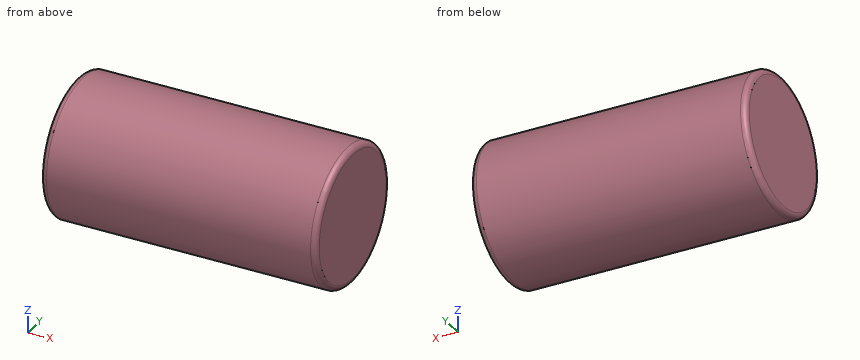
```python
from build123d import *

# Parameters (mm, degrees)
F0_R          = 76.09774
F1_DEPTH      = 152.4
F1_DEPTH_BACK = 152.4
F2_R          = 6.35
F3_R          = 6.35


with BuildPart() as f1:
    # F0 (on Right) → F1 (new body, two sides)
    with BuildSketch(Plane.YZ) as f1_sk:
        Circle(F0_R)
    extrude(amount=F1_DEPTH)
    extrude(f1_sk.sketch, amount=-F1_DEPTH_BACK)

    # F2
    f2_edges = [f1.edges().sort_by_distance(p)[0] for p in [
        (152.4, -76.09774, 0),
    ]]
    fillet(f2_edges, radius=F2_R)

    # F3
    f3_edges = [f1.edges().sort_by_distance(p)[0] for p in [
        (-152.4, -76.09774, 0),
    ]]
    fillet(f3_edges, radius=F3_R)


solid = f1.part
```
Can you work these out from the model? Positions are in its coordinate system, mm. Round coordinates to 2 decimals unless told otherwise and drop trailing zeros. Loops run counter-clockwise (first coordinate to the right, second up) from the corner with the lowest first, then second, coordinate; pieces in that order, holes last. Notation, with made-up numbers: M 73.25,53 L 101.25,53 A8 cw 101.25,63 Z; hole C 87.5,65.25 d8. An arc over 180 degrees is marked long. Answer as a JSON object with one key per item and string values. Group by question number.
Q1. Please list where these lines run through material, in increasing order: L1, parallel to Y at x = 84, z = -2; L2, parallel to Z at x = 37, y = 51.
Q2. Imagine slicing it at A-A, the plane x = -111.5. Please give me the cut outline in (y, z), then the cut area to 3 significant figures.
Q3. Will these pins go through, and if not, where does the flat tip stop? pin 1 (3 mm diameter, centred on x = 26.5, z = 39, fed in from -Y); pin 2 (1 mm diameter, centred on x = 118, z = -42.5, fed in from -Y); pin 3 (4 mm diameter, centred on x = 18.5, z = -37.5, fed in from -Y).
Findings:
{
 "1": {"L1": "y = -76.07 to 76.07", "L2": "z = -56.48 to 56.48"},
 "2": {"outline": "C 0,0 d152.2", "area": "18,200 mm2"},
 "3": {"pin 1": "stops at y = -66.22", "pin 2": "stops at y = -63.46", "pin 3": "stops at y = -67.31"}
}
